Design review of the part built by this model. Coordinates are the model's own, in mm. Give positions to 0.01 mm unless a question says otherwise; leave off trailing zeros. Loops run counter-clockwise (first coordinate to the right, second up) from the corner with the lowest first, then second, coordinate; pieces in that order, holes last.
from build123d import *

# Parameters (mm, degrees)
SKETCH1_R           = 1.025
BOSS_EXTRUDE1_DEPTH = 1.3
SKETCH2_W           = 2.45
SKETCH2_H           = 4.7
BOSS_EXTRUDE2_DEPTH = 2
SKETCH3_W           = 2.378127828
SKETCH3_H           = 0.99144163
BOSS_EXTRUDE3_DEPTH = 1.4


with BuildPart() as part:
    # Sketch1 → Boss-Extrude1 (new body)
    with BuildSketch(Plane(origin=(0, 0, 0), x_dir=(1, 0, 0), z_dir=(0, 1, 0))):
        with BuildLine():
            Line((3, 0), (26, 0))
            ThreePointArc((26, 0), (28.121320344, 0.878679656), (29, 3))
            Line((29, 3), (29, 26))
            ThreePointArc((29, 26), (28.121320344, 28.121320344), (26, 29))
            Line((26, 29), (3, 29))
            ThreePointArc((3, 29), (0.878679656, 28.121320344), (0, 26))
            Line((0, 26), (0, 3))
            ThreePointArc((0, 3), (0.878679656, 0.878679656), (3, 0))
        make_face()
        with Locations((4.5, 24.5)):
            Circle(SKETCH1_R, mode=Mode.SUBTRACT)
        with Locations((24.5, 24.5)):
            Circle(SKETCH1_R, mode=Mode.SUBTRACT)
        with Locations((24.5, 4.5)):
            Circle(SKETCH1_R, mode=Mode.SUBTRACT)
        with Locations((4.5, 4.5)):
            Circle(SKETCH1_R, mode=Mode.SUBTRACT)
    extrude(amount=BOSS_EXTRUDE1_DEPTH)

    # Sketch2 → Boss-Extrude2 (add)
    with BuildSketch(Plane(origin=(0, 1.3, 0), x_dir=(1, 0, 0), z_dir=(0, 1, 0))):
        with Locations((27.511966954, 19.85)):
            Rectangle(SKETCH2_W, SKETCH2_H)
        with Locations((27.511966954, 9.15)):
            Rectangle(SKETCH2_W, SKETCH2_H)
    extrude(amount=BOSS_EXTRUDE2_DEPTH)

    # Sketch3 → Boss-Extrude3 (add)
    with BuildSketch(Plane(origin=(28.736966954, 0, 0), x_dir=(0, 0, -1), z_dir=(1, 0, 0))):
        with Locations((9.15, 2.3)):
            Rectangle(SKETCH3_W, SKETCH3_H)
        with Locations((19.85, 2.3)):
            Rectangle(SKETCH3_W, SKETCH3_H)
    extrude(amount=BOSS_EXTRUDE3_DEPTH)


solid = part.part
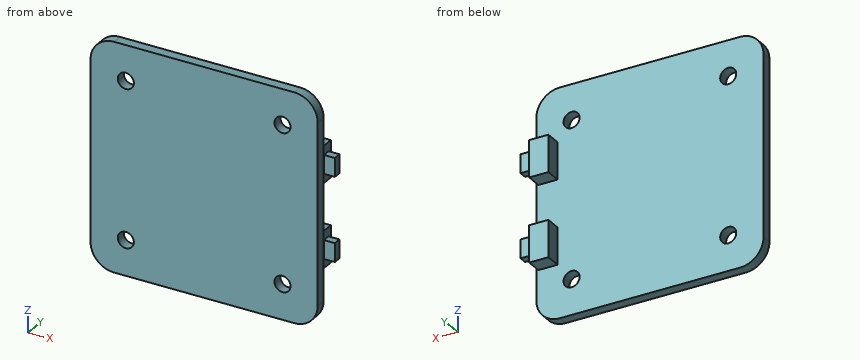
Q1. Insertion check: pin 1 (0.7 mm diameter, centred on x = 29.5, z = -9.5, fed in from +Y); pin 2 (5 mm diameter, centred on x = 15.5, z = -22.5, fed in from +Y); pin 3 (1.1 mm diameter, centred on x = 29.5, y = 2.5, fed in from +Z); pin 4 (1.8 mm diameter, centred on x = 4.5, z = -4.5, fed in from +Y). Each pin has a flat end and moves straight along its axis. Give the tip position at first contact, or say it passes through.
Results:
pin 1: stops at y = 2.8
pin 2: stops at y = 1.3
pin 3: stops at z = -7.96
pin 4: passes through
Q2. Take a section at C-C (y = 2.15). Give the boundary of the cut face in (x, z), plus the area to 3 significant figures.
Results:
outline: (26.29, -22.2) - (28.74, -22.2) - (28.74, -21.04) - (30.14, -21.04) - (30.14, -18.66) - (28.74, -18.66) - (28.74, -17.5) - (26.29, -17.5) - close; (26.29, -11.5) - (28.74, -11.5) - (28.74, -10.34) - (30.14, -10.34) - (30.14, -7.96) - (28.74, -7.96) - (28.74, -6.8) - (26.29, -6.8) - close
area: 29.7 mm2
Q3. Wall thickness on line 1 (X direction, y = 0.75, z = -4.5) (3 decimals); line 2 (Z direction, x = 24.5, y = 0.55) (3 decimals); line 3 (Y direction, x = 12, z = -17.5): over which ranges is each line inside the solid? List them lowest first.
Results:
line 1: x = 0 to 3.475, 5.525 to 23.475, 25.525 to 29
line 2: z = -29 to -25.525, -23.475 to -5.525, -3.475 to 0
line 3: y = 0 to 1.3
Q4. Take a section at D-D (z = -10.75). Give the boundary of the cut face in (x, y).
Results:
outline: (0, 0) - (29, 0) - (29, 1.3) - (28.74, 1.3) - (28.74, 3.3) - (26.29, 3.3) - (26.29, 1.3) - (0, 1.3) - close
Q5. Take a section at B-B (z = -24.5). Give the boundary of the cut face in (x, y) (3 decimals), plus the area to 3 significant figures.
Results:
outline: (0, 0) - (3.475, 0) - (3.475, 1.3) - (0, 1.3) - close; (5.525, 0) - (23.475, 0) - (23.475, 1.3) - (5.525, 1.3) - close; (25.525, 0) - (29, 0) - (29, 1.3) - (25.525, 1.3) - close
area: 32.4 mm2
Q6. Take a section at A-A (x = 24.5). Give the boundary of the cut face in (y, z) (3 decimals).
Results:
outline: (0, -29) - (1.3, -29) - (1.3, -25.525) - (0, -25.525) - close; (0, -23.475) - (1.3, -23.475) - (1.3, -5.525) - (0, -5.525) - close; (0, -3.475) - (1.3, -3.475) - (1.3, 0) - (0, 0) - close
